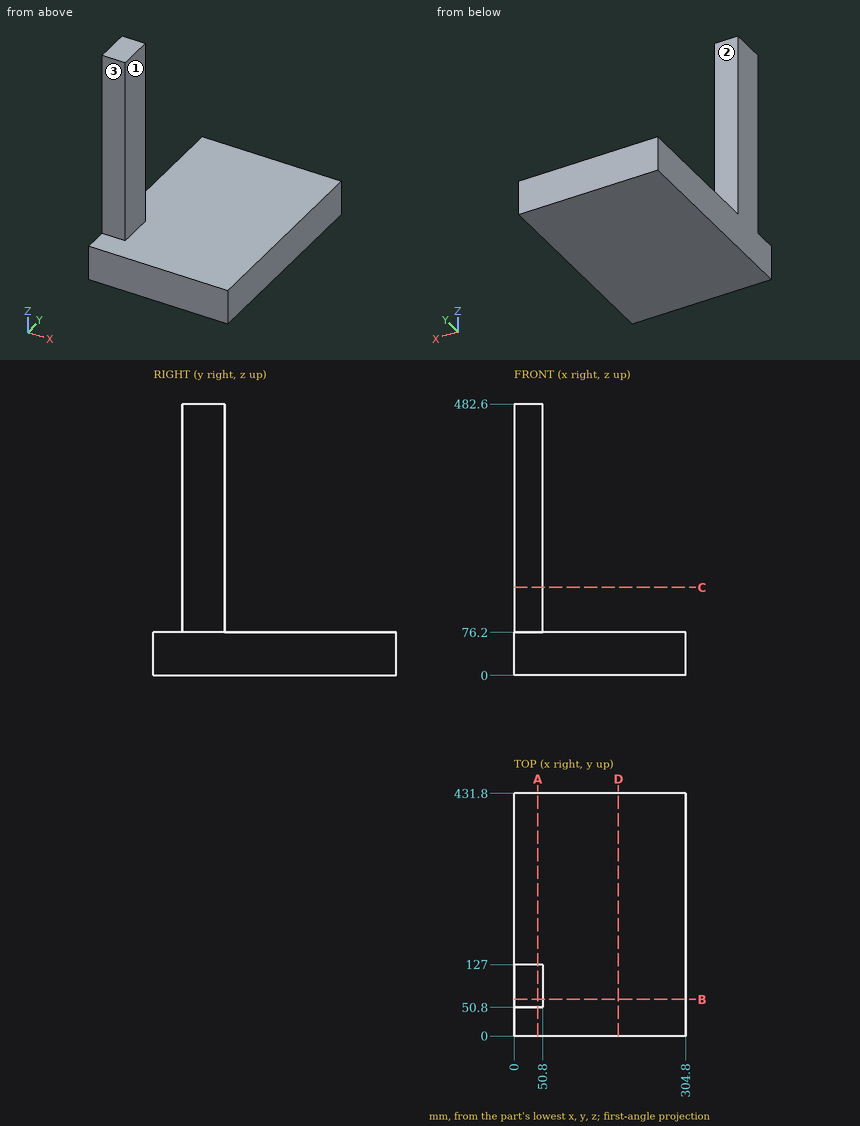
Verification items for this drawing (mm, ordinates from the low corner). A direction names the side the tool comes from. Round coordinates to 2 decimals unless told otherwise and drop trailing zeros. Write each loop counter-clockwise with the first axis right and the second up, starting at its lowest first coordinate (ties: lowest second). Pieces come first, ordered by that corner, then holes. Notation, with made-up numbers: M -11,-21.75 L 13,-21.75 A35 cw 13,16.25 Z; hole C 44.5,62 d3. An arc over 180 degrees is marked long. Write item = value, one per line. Start each with the question number.
1. Section check D-D, the plane x = 185.5. Record the cut outline in (y, z), then the cut area to 3 significant figures.
2. Section check B-B, the plane y = 65. Record the cut outline in (x, z), then the cut area to 3 significant figures.
3. Scan lines: line 1 (Z direction, x = 241, y = 309); line 2 (X direction, y = 54, z = 433). Record each from-to range of solid material in increasing order. Write a range as [from, to].
4. Section check C-C, the plane z = 156.5. Record the cut outline in (x, y), then the cut area to 3 significant figures.
5. Gauge pin test, flat ends, axial feed: pin 1 (15 mm diameter, centred on x = 18.5, z = 213, fed in from -Y); pin 2 (8 mm diameter, centred on x = 123, y = 211, fed in from +Z). Record the tip position at first contact, or that the pin passes through.
6. Tool access check on the marked faces 1, 2 and 3. Record the directions out of +Z, -Z, +X, -X, +Y, -Y that give a thin tool (end or side, any length) a straight path to the whole face; none if there is none.
7. Section check A-A, the plane x = 42. Record the cut outline in (y, z).
Results found:
q1.outline = M 0,0 L 431.8,0 L 431.8,76.2 L 0,76.2 Z
q1.area = 32,900 mm^2
q2.outline = M 0,0 L 304.8,0 L 304.8,76.2 L 50.8,76.2 L 50.8,482.6 L 0,482.6 Z
q2.area = 43,900 mm^2
q3.line_1 = [0, 76.2]
q3.line_2 = [0, 50.8]
q4.outline = M 0,50.8 L 50.8,50.8 L 50.8,127 L 0,127 Z
q4.area = 3,870 mm^2
q5.pin_1 = 50.8
q5.pin_2 = 76.2
q6.face_1 = +Z, +X, +Y, -Y
q6.face_2 = +Z, +X, -X, +Y
q6.face_3 = +Z, +X, -X, -Y
q7.outline = M 0,0 L 431.8,0 L 431.8,76.2 L 127,76.2 L 127,482.6 L 50.8,482.6 L 50.8,76.2 L 0,76.2 Z
